Part model, mm, in its own coordinate system. Round coordinates to 2 decimals unless told otherwise and drop trailing zeros. Order: outer loops, then holes, each group sorted by start corner. A loop starts at its lowest first (then second) coordinate and runs counter-clockwise, first axis right, second up. Notation, with made-up numbers: (-15, 22) - (40, 22) arc R9 ccw to (40, 30) - close; hole circle Ø9 at (85.5, -4). An arc over 180 degrees is marked (long way). Answer as a JSON object with one key per item and string values.
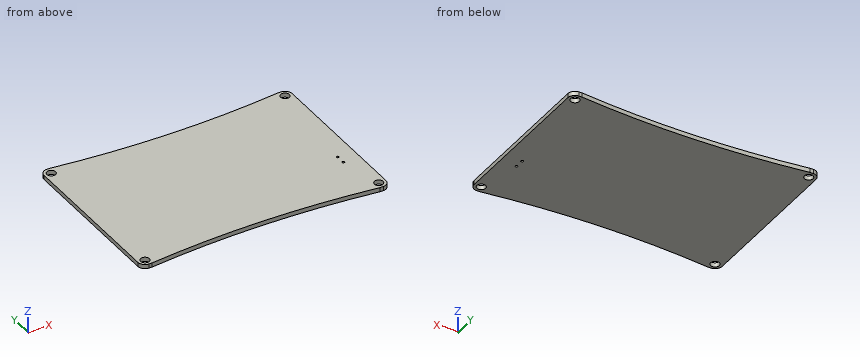
```python
from build123d import *

# Parameters (mm, degrees)
BOARD_OUTLINE_DEPTH = 1.62
SKETCH2_R           = 0.45
NPTH_DEPTH          = 117.618264864
SKETCH3_R           = 1.65
PTH_DEPTH           = 117.618264864


with BuildPart() as part:
    # Sketch1 → Board_Outline (new body)
    with BuildSketch(Plane.XY):
        with BuildLine():
            Line((2.54, 62.89), (2.54, 3.15))
            ThreePointArc((2.54, 3.15), (3.322492676, 1.392492676), (5.08, 0.61))
            Line((5.08, 0.61), (6.35, 0.61))
            ThreePointArc((6.35, 0.61), (49.53, 3.251001938), (92.71, 0.61))
            Line((92.71, 0.61), (93.98, 0.61))
            ThreePointArc((93.98, 0.61), (95.737507324, 1.392492676), (96.52, 3.15))
            Line((96.52, 3.15), (96.52, 62.89))
            ThreePointArc((96.52, 62.89), (95.737507324, 64.647507324), (93.98, 65.43))
            Line((93.98, 65.43), (92.71, 65.43))
            ThreePointArc((92.71, 65.43), (49.53, 62.788998062), (6.35, 65.43))
            Line((6.35, 65.43), (5.08, 65.43))
            ThreePointArc((5.08, 65.43), (3.322492676, 64.647507324), (2.54, 62.89))
        make_face()
    extrude(amount=BOARD_OUTLINE_DEPTH)

    # Sketch2 → NPTH (cut, through all)
    with BuildSketch(Plane.XY):
        with Locations((90.17, 23.09)):
            Circle(SKETCH2_R)
        with Locations((90.17, 19.59)):
            Circle(SKETCH2_R)
    extrude(amount=NPTH_DEPTH, mode=Mode.SUBTRACT)

    # Sketch3 → PTH (cut, through all)
    with BuildSketch(Plane.XY):
        with Locations((93.83, 3.28)):
            Circle(SKETCH3_R)
        with Locations((5.23, 3.28)):
            Circle(SKETCH3_R)
        with Locations((5.23, 62.76)):
            Circle(SKETCH3_R)
        with Locations((93.83, 62.76)):
            Circle(SKETCH3_R)
    extrude(amount=PTH_DEPTH, mode=Mode.SUBTRACT)


solid = part.part
```
Item 1: Probe L1, parallel to Y at x = 5.23, z = 1.05; L2, parallel to X at y = 23.09, z = 0.5; L3, parallel to X at y = 4.5, z = 0.15. List the from-to ranges inside material, lowest first. Write a range as from..to.
Taken from the geometry:
{"L1": "0.61..1.63, 4.93..61.11, 64.41..65.43", "L2": "2.54..89.72, 90.62..96.52", "L3": "2.54..4.12, 6.34..92.72, 94.94..96.52"}
Item 2: Cut at C-C (x = 83). Write the cut outline in (y, z), plus the area to 3 significant figures.
Taken from the geometry:
{"outline": "(1.67, 0) - (64.37, 0) - (64.37, 1.62) - (1.67, 1.62) - close", "area": "102 mm2"}
Item 3: Cut at B-B (x = 39). Write the cut outline in (y, z), plus the area to 3 significant figures.
Taken from the geometry:
{"outline": "(3.09, 0) - (62.95, 0) - (62.95, 1.62) - (3.09, 1.62) - close", "area": "97.0 mm2"}
Item 4: Cut at A-A (z = 1.2). Write the cut outline in (x, y).
Taken from the geometry:
{"outline": "(2.54, 3.15) arc R2.68 ccw to (5.08, 0.61) - (6.35, 0.61) arc R354.31 cw to (92.71, 0.61) - (93.98, 0.61) arc R2.68 ccw to (96.52, 3.15) - (96.52, 62.89) arc R2.68 ccw to (93.98, 65.43) - (92.71, 65.43) arc R354.31 cw to (6.35, 65.43) - (5.08, 65.43) arc R2.68 ccw to (2.54, 62.89) - close; hole circle Ø3.3 at (5.23, 3.28); hole circle Ø3.3 at (5.23, 62.76); hole circle Ø0.9 at (90.17, 19.59); hole circle Ø0.9 at (90.17, 23.09); hole circle Ø3.3 at (93.83, 3.28); hole circle Ø3.3 at (93.83, 62.76)"}
